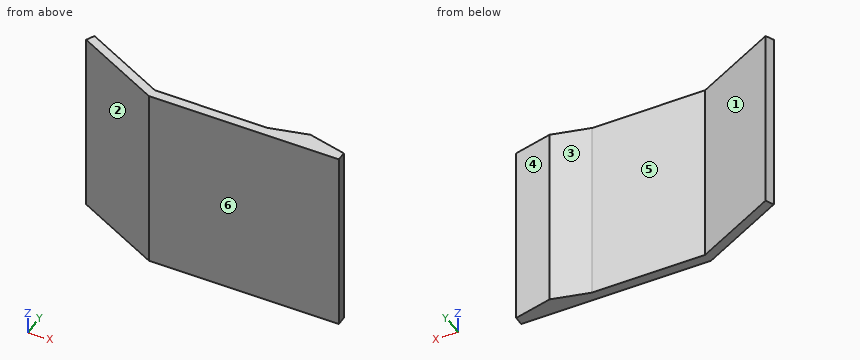
```python
from build123d import *

# Parameters (mm, degrees)
RESSALTO_EXTRUS_O1_DEPTH = 400


with BuildPart() as part:
    # Esboço1 → Ressalto-extrusão1 (new body)
    with BuildSketch(Plane.XY):
        Polygon((8.601413754, 16.881224995), (0, 0), (400, 0), (400, 20), (240, 20), (2.480473166, 20), align=None)
        Polygon((-179.558563965, 91.489658015), (0, 0), (0, 20), (2.480473166, 20), (-170.957150212, 108.37088301), align=None)
        Polygon((0, 20), (0, 0), (8.601413754, 16.881224995), (2.480473166, 20), align=None)
        Polygon((240, 20), (400, 20), (320, 39.206300726), align=None)
    extrude(amount=RESSALTO_EXTRUS_O1_DEPTH)


solid = part.part
```
Source: CAD feature listing. Evaluate the final solid. Frame: model axes, mm. Face numbers are marked on the shaded views. A direction names the side the tool comes from. Give positions to 0.01 mm unless a question says otherwise; leave off trailing zeros. Write each loop counter-clockwise with the first axis right and the second up, starting at its lowest first coordinate (ties: lowest second). Pieces come first, ordered by that corner, then holes.
1. Section query B-B (y = 33). Return the cut outline in (x, z).
2. Pull-direction query (X, two-part tool) for the marked faces 3, 4, 5 and 6; classes: +X half, -X half, draft (parallel to the pull), parting line (faces both ways), or undercut.
3. Material intervals for line 1 along Y through (x, z) = (69.5, 200.5); line 2 along Y through (x, z) = (240.5, 58); line 3 along X through (y, z) = (98, 233.5), sorted ascending.
4. First-contact query: pin 1 (2 mm diameter, centred on x = 298.5, z = 206.5, fed in from +Y); pin 2 (5 mm diameter, centred on y = 21, z = 322.5, fed in from -X); pin 3 (8 mm diameter, centred on y = 49, z = 194.5, fed in from +X); pin 4 (2 mm diameter, centred on x = 55.5, z = 300.5, fed in from -Y). Flat tips, straight axial feed; report the tip coordinate or a pass-through.
5. Section query C-C (x = 60.5). Return the cut outline in (y, z).
6. Section query D-D (y = 62.5). Return the cut outline in (x, z).
7. Section query A-A (z = 69.5). Return the cut outline in (x, y), then the cut area to 3 significant figures.
8. Access query for the marked faces 1 and 2. Directions: +Z, -Z, +X, -X, +Y, -Y. A direction counts if a zero-diameter tool reaches every point of the face in a straight line with its end or side. Return the directions, or none.
Output values:
1. outline: (-64.77, 0) - (-23.03, 0) - (-23.03, 400) - (-64.77, 400) - close; (294.15, 0) - (345.85, 0) - (345.85, 400) - (294.15, 400) - close
2. face 3: undercut
2. face 4: +X half
2. face 5: undercut
2. face 6: draft
3. line 1: y = 0 to 20
3. line 2: y = 0 to 20.12
3. line 3: x = -176.24 to -150.6
4. pin 1: stops at y = 34.28
4. pin 2: stops at x = -46.12
4. pin 3: stops at x = -46.58
4. pin 4: stops at y = 0
5. outline: (0, 0) - (20, 0) - (20, 400) - (0, 400) - close
6. outline: (-122.66, 0) - (-80.93, 0) - (-80.93, 400) - (-122.66, 400) - close
7. outline: (-179.56, 91.49) - (0, 0) - (400, 0) - (400, 20) - (320, 39.21) - (240, 20) - (2.48, 20) - (-170.96, 108.37) - close
7. area: 13,300 mm2
8. face 1: +Z, -Z, +Y
8. face 2: +Z, -Z, -X, -Y
